Could you check a few things on this model? Use its own coordinates, in mm. Face numbers are marked on the shaded views. Give positions to 0.01 mm unless a question says otherwise; leave off trailing zeros. Order: outer loops, then holes, each group sorted by start corner. A loop starts at its lowest first (then second) coordinate and runs counter-clockwise, first axis right, second up. Notation, with made-up numbers: (23.5, -39.5) - (56.5, -39.5) arc R21 cw to (56.5, -31.5) - close; hole circle Ø9 at (59, 24.25). An arc over 180 degrees is marked (long way). Put each result on its own line as item: value.
from build123d import *


with BuildPart() as part:
    # Sketch1 → Revolve1 (revolve)
    with BuildSketch(Plane.XY, mode=Mode.PRIVATE) as revolve1_sk:
        with BuildLine():
            Line((-37.809513487, -40), (-32.425741253, -40))
            Line((-32.425741253, -40), (-32.425741253, -38))
            Line((-32.425741253, -38), (-37.809513487, -38))
            ThreePointArc((-37.809513487, -38), (-37.908222233, -38.083981776), (-37.841136263, -38.19486833))
            Line((-37.841136263, -38.19486833), (-35.994951232, -38.81026334))
            ThreePointArc((-35.994951232, -38.81026334), (-35.858196785, -39), (-35.994951232, -39.18973666))
            Line((-35.994951232, -39.18973666), (-37.841136263, -39.80513167))
            ThreePointArc((-37.841136263, -39.80513167), (-37.908222233, -39.916018224), (-37.809513487, -40))
        make_face()
    revolve(revolve1_sk.sketch.rotate(Axis((-83.208746897, 0, 0), (1, 0, 0)), 270), axis=Axis((-83.208746897, 0, 0), (1, 0, 0)))


solid = part.part
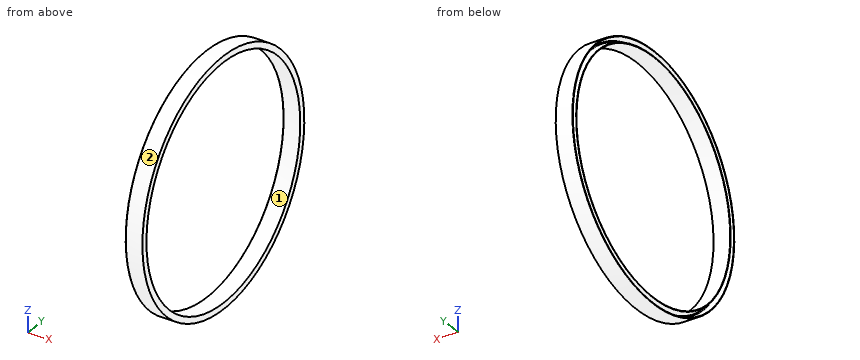
1) Suppose I cut it at A-A, the plane y = 0. List the corners of the cut face in (x, z) for me.
Filled in:
outline: (-37.84, -39.81) arc R0.1 ccw to (-37.81, -40) - (-32.43, -40) - (-32.43, -38) - (-37.81, -38) arc R0.1 ccw to (-37.84, -38.19) - (-35.99, -38.81) arc R0.2 cw to (-35.99, -39.19) - close; (-37.84, 38.19) arc R0.1 ccw to (-37.81, 38) - (-32.43, 38) - (-32.43, 40) - (-37.81, 40) arc R0.1 ccw to (-37.84, 39.81) - (-35.99, 39.19) arc R0.2 cw to (-35.99, 38.81) - close
2) I'm going to push flat-ended pins straight in: pin 1 (2 mm diameter, centred on x = -36, z = -7, fed in from +Y); pin 2 (1 mm diameter, centred on x = -37, z = -31.5, fed in from +Y); pin 3 (3 mm diameter, centred on x = -37, y = -16, fed in from +Z). Where does each tip first touch, or does it pass through?
Filled in:
pin 1: stops at y = 39.55
pin 2: stops at y = 25.28
pin 3: stops at z = 37.28
3) We'd pull the mould along Z, two halves only. Please class the marked faces 1 and 2: pulls with the +Z half, pulls with the -Z half, needs draft (parallel to the pull), parting line crosses it, or undercut.
Filled in:
face 1: undercut
face 2: parting line crosses it
4) If I drill on line 1 (Y direction, x = -35.3, z = 0); line 2 (Y direction, x = -37.35, z = -8); line 3 (Y direction, x = -36.2, z = -12), over which ranges is the centre line in solid material (lowest first)? Write a range as [from, to].
Filled in:
line 1: y = [-40, -38], [38, 40]
line 2: y = [-39.19, -38.83], [-37.52, -37.15], [37.15, 37.52], [38.83, 39.19]
line 3: y = [-38.16, -37.38], [-36.84, -36.06], [36.06, 36.84], [37.38, 38.16]
5) Suppose I cut it at C-C, the plane x = -33.6. List the corners of the cut face in (y, z) for me, and give its area (3 significant figures).
Filled in:
outline: circle Ø80 at (0, 0); hole circle Ø76 at (0, 0)
area: 490 mm^2
